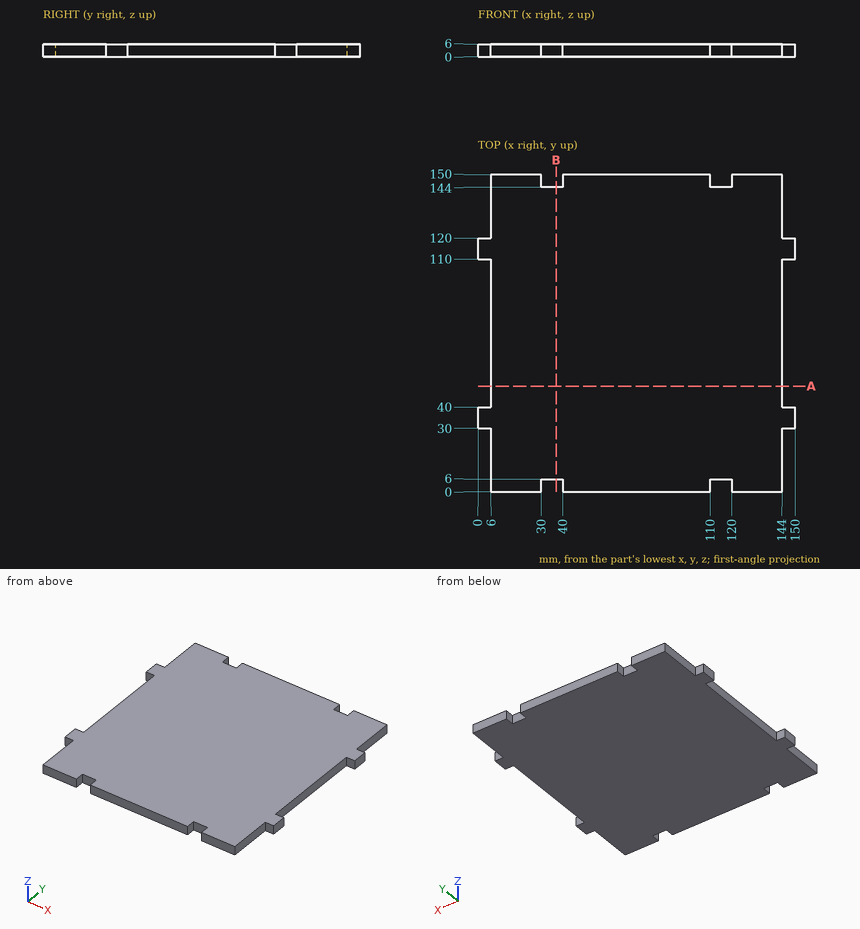
Geometry: see drawing. Coordinates: mm, zero at the bounding-box minimum. Give positions to 0.01 mm unless a question says otherwise; leave off trailing zeros. Write each loop counter-clockwise with the first axis right and the second up, starting at its lowest first coordinate (ties: lowest second). Pieces come first, ordered by that corner, then holes. Notation, with made-up numbers: M 58,61.25 L 63,61.25 A11 ccw 63,71.25 Z; hole C -30,51 d5. An arc over 180 degrees is marked long. Answer in a Markdown table with one row per item. Add a question column.
(1) Ray query, line 1 (X direction, y = 24.5, z = 4.1). Return the intervals inside material, ascending.
(2) Section A-A on y = 50. Return loops of the section in (x, z).
(3) First-contact query: pin 1 (1.8 mm diameter, centred on y = 132.5, z = 2, fed in from +X); pin 2 (1.5 mm diameter, centred on y = 64, z = 3, fed in from -X); pin 3 (3 mm diameter, centred on x = 117, z = 3, fed in from +Y). Flat tips, straight axial feed; report the tip coordinate or a pass-through.
Result set:
| question | item | result |
|---|---|---|
| 1 | line 1 | x = 6 to 144 |
| 2 | outline | M 6,0 L 144,0 L 144,6 L 6,6 Z |
| 3 | pin 1 | stops at x = 144 |
| 3 | pin 2 | stops at x = 6 |
| 3 | pin 3 | stops at y = 144 |
